Verification items for the finished model (mm, model axes). Face numbers are marked on the shaded views. A direction names the side the tool comes from. Round coordinates to 2 decimals unless told otherwise and drop trailing zeros. Write each loop counter-clockwise with the first axis right and the second up, starting at its lowest first coordinate (ties: lowest second). Pieces come first, ordered by that corner, then holes. Notation, with made-up numbers: M -28,9 L 22,9 A14 ccw 22,17 Z; hole C 68,-35 d9. An arc over 180 degrees is marked long. Write each question's results on one line, items separated by ' | '.
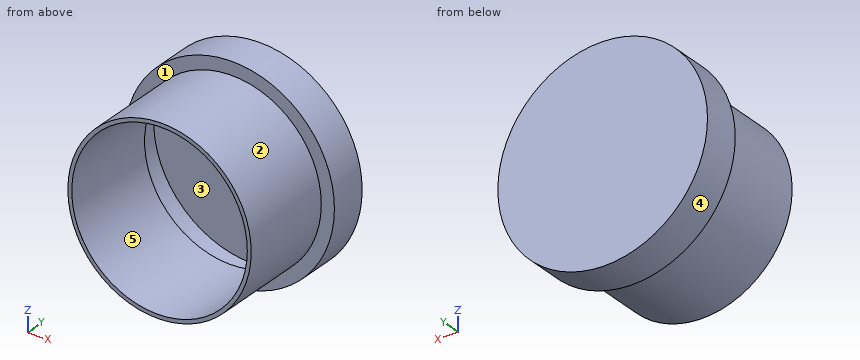
from build123d import *

# Parameters (mm, degrees)
F0_R     = 67.9912041861
F1_DEPTH = 25.4
F2_R     = 59.4709809198
F3_DEPTH = 89.535
F4_T     = -2.54


with BuildPart() as f1:
    # F0 (on Front) → F1 (new body)
    with BuildSketch(Plane.XZ):
        Circle(F0_R)
    extrude(amount=F1_DEPTH)

    # F2 (on Front) → F3 (join)
    with BuildSketch(Plane.XZ):
        Circle(F2_R)
    extrude(amount=F3_DEPTH)

    # F4
    f4_openings = [f1.faces().sort_by_distance(p)[0] for p in [
        (0, -89.535, 0),
    ]]
    offset(amount=F4_T, openings=f4_openings, kind=Kind.INTERSECTION)


solid = f1.part
1) Sectioned sample at A-A, the plane x = 0. Record the cut outline in (y, z) (3 decimals), and give its area (3 significant figures).
Calculated:
outline: M -89.535,-59.471 L -25.4,-59.471 L -25.4,-67.991 L 0,-67.991 L 0,67.991 L -25.4,67.991 L -25.4,59.471 L -89.535,59.471 L -89.535,56.931 L -22.86,56.931 L -22.86,65.451 L -2.54,65.451 L -2.54,-65.451 L -22.86,-65.451 L -22.86,-56.931 L -89.535,-56.931 Z | area: 831 mm²
2) Depth check by flat-ended pin: P1, Ø6, axis at x = -22, y = -25, coming from the -Z side; P2, Ø6, axis at x = 46, y = -16, coming from the -Z side; P3, Ø3, axis at y = -12, z = -29.5, coming from the +X side. Enter the tip coordinate at first touch or a pass-through.
Calculated:
P1: stops at z = -65.28 | P2: stops at z = -52.67 | P3: stops at x = 61.96
3) Sectioned sample at D-D, the plane y = -73. Record the cut outline in (x, z), and give its area (3 significant figures).
Calculated:
outline: C 0,0 d118.94; hole C 0,0 d113.86 | area: 929 mm²
4) Sectioned sample at C-C, the plane y = -20.5. Record the cut outline in (x, z).
Calculated:
outline: C 0,0 d135.98; hole C 0,0 d130.9
5) Access from +Z, -Z, +X, -X, +Y, -Y to the whole of each face (thin tool, end or side, straight path). Record for the marked faces 4 and 5.
Calculated:
face 4: +Y, -Y | face 5: -Y
6) Sectioned sample at B-B, the plane z = 0. Record the cut outline in (x, y) (3 decimals), and give its area (3 significant figures).
Calculated:
outline: M -67.991,-25.4 L -59.471,-25.4 L -59.471,-89.535 L -56.931,-89.535 L -56.931,-22.86 L -65.451,-22.86 L -65.451,-2.54 L 65.451,-2.54 L 65.451,-22.86 L 56.931,-22.86 L 56.931,-89.535 L 59.471,-89.535 L 59.471,-25.4 L 67.991,-25.4 L 67.991,0 L -67.991,0 Z | area: 831 mm²
7) Material ranges on line 1 (Y direction, x = 46, z = -45.5); line 2 (X direction, y = -59.5, z = 0); line 3 (Z direction, x = 0, y = -18.75), recorded low to high. Write a range as [from, to].
Calculated:
line 1: y = [-25.4, -22.86], [-2.54, 0] | line 2: x = [-59.47, -56.93], [56.93, 59.47] | line 3: z = [-67.99, -65.45], [65.45, 67.99]
8) Draft check along Z on the marked faces 1, 2 and 3. Enter one of: pulls with the +Z half, pulls with the -Z half, needs draft (parallel to the pull), parting line crosses it, or undercut.
Calculated:
face 1: needs draft | face 2: parting line crosses it | face 3: undercut
